Build history of the part. All positions in model axes, mm. A direction names the side the tool comes from. Round coordinates to 2 decimals unless told otherwise and drop trailing zeros. Loops run counter-clockwise (first coordinate to the right, second up) from the corner with the lowest first, then second, coordinate; pieces in that order, holes last. Notation, with made-up numbers: M 58,0.5 L 71,0.5 A17 ccw 71,33.5 Z; hole C -15,-33.75 d4. An arc over 180 degrees is marked long. One line per item, written item: value.
```python
from build123d import *

# Parameters (mm, degrees)
SKETCH1_R           = 38.1
SKETCH1_R_2         = 6.35
BOSS_EXTRUDE1_DEPTH = 2.54
SKETCH2_R           = 8.89
SKETCH2_R_2         = 6.35
BOSS_EXTRUDE2_DEPTH = 6.35
SKETCH5_R           = 38.1
SKETCH5_R_2         = 30.48
BOSS_EXTRUDE3_DEPTH = 2.54
SKETCH6_R           = 38.1
SKETCH6_R_2         = 35.56
BOSS_EXTRUDE4_DEPTH = 6.35


with BuildPart() as part:
    # Sketch1 → Boss-Extrude1 (new body)
    with BuildSketch(Plane(origin=(0, 0, 0), x_dir=(1, 0, 0), z_dir=(0, 1, 0))):
        with Locations(Location((0, 0, 0), (0, 0, 270))):
            Circle(SKETCH1_R)
        with Locations(Location((0, 0, 0), (0, 0, 270))):
            Circle(SKETCH1_R_2, mode=Mode.SUBTRACT)
    extrude(amount=BOSS_EXTRUDE1_DEPTH)

    # Sketch2 → Boss-Extrude2 (add)
    with BuildSketch(Plane(origin=(0, 2.54, 0), x_dir=(1, 0, 0), z_dir=(0, 1, 0))):
        with Locations(Location((0, 0, 0), (0, 0, 270))):
            Circle(SKETCH2_R)
        with Locations(Location((0, 0, 0), (0, 0, 270))):
            Circle(SKETCH2_R_2, mode=Mode.SUBTRACT)
    extrude(amount=BOSS_EXTRUDE2_DEPTH)

    # Sketch5 → Boss-Extrude3 (add)
    with BuildSketch(Plane(origin=(0, 2.54, 0), x_dir=(1, 0, 0), z_dir=(0, 1, 0))):
        with Locations(Location((0, 0, 0), (0, 0, 270))):
            Circle(SKETCH5_R)
        with Locations(Location((0, 0, 0), (0, 0, 270))):
            Circle(SKETCH5_R_2, mode=Mode.SUBTRACT)
    extrude(amount=BOSS_EXTRUDE3_DEPTH)

    # Sketch6 → Boss-Extrude4 (add)
    with BuildSketch(Plane(origin=(0, 5.08, 0), x_dir=(1, 0, 0), z_dir=(0, 1, 0))):
        with Locations(Location((0, 0, 0), (0, 0, 270))):
            Circle(SKETCH6_R)
        with Locations(Location((0, 0, 0), (0, 0, 270))):
            Circle(SKETCH6_R_2, mode=Mode.SUBTRACT)
    extrude(amount=BOSS_EXTRUDE4_DEPTH)


solid = part.part
```
Item 1: Slice it at D-D, the plane y = 1.25. Give the cut face in (x, z), and give its area (3 significant figures).
Check values:
outline: C 0,0 d76.2; hole C 0,0 d12.7
area: 4,430 mm2
Item 2: Pull direction X, two halves, no side cores. Call faces 1 (the face through (-23.183, 5.635, -30.235)), 2 (the face through (30.22, 3.79, -3.97)), 3 (the face through (11, 11.43, 34)): pulls with the +X half, pulls with the -X half, needs draft (parallel to the pull), parting line crosses it, or undercut.
Check values:
face 1: parting line crosses it
face 2: undercut
face 3: needs draft
Item 3: Drop flat-ended pins along their axis: P1, Ø14.5, axis at x = 0, z = 0, coming from the +Y side; P2, Ø2, axis at x = -1.5, z = 10, coming from the +Y side; P3, Ø12, axis at x = 17.5, z = 20, coming from the +Y side. Give the stop position or say it passes through.
Check values:
P1: stops at y = 8.89
P2: stops at y = 2.54
P3: stops at y = 5.08
Item 4: Slice it at A-A, the plane x = 0. Give the cut face in (y, z).
Check values:
outline: M 0,-38.1 L 11.43,-38.1 L 11.43,-35.56 L 5.08,-35.56 L 5.08,-30.48 L 2.54,-30.48 L 2.54,-8.89 L 8.89,-8.89 L 8.89,-6.35 L 0,-6.35 Z; M 0,6.35 L 8.89,6.35 L 8.89,8.89 L 2.54,8.89 L 2.54,30.48 L 5.08,30.48 L 5.08,35.56 L 11.43,35.56 L 11.43,38.1 L 0,38.1 Z
Item 5: Wall check: line 1 along X through (y, z) = (8.25, 0); line 2 along X through (y, z) = (3.35, 0); line 3 along X through (y, z) = (9.25, 0). Give the ranges that are in metal, low to high.
Check values:
line 1: x = -38.1 to -35.56, -8.89 to -6.35, 6.35 to 8.89, 35.56 to 38.1
line 2: x = -38.1 to -30.48, -8.89 to -6.35, 6.35 to 8.89, 30.48 to 38.1
line 3: x = -38.1 to -35.56, 35.56 to 38.1
Item 6: Slice it at C-C, the plane y = 8. Give the cut face in (x, z).
Check values:
outline: C 0,0 d76.2; C 0,0 d17.78; hole C 0,0 d71.12; hole C 0,0 d12.7
Item 7: Which spindle directions (+Z, -Z, +X, -X, +Y, -Y) get a long thin tool onto all of the face, cutting with end or side? Do faces 4 (the face through (-8.68, 5.67, -1.93)), 5 (the face through (-3.86, 4.38, -5.04)). Say none if no direction does.
Check values:
face 4: +Y
face 5: +Y, -Y
Item 8: Slice it at B-B, the plane z = 0. Give the cut face in (x, y), and give its area (3 significant figures).
Check values:
outline: M -38.1,0 L -6.35,0 L -6.35,8.89 L -8.89,8.89 L -8.89,2.54 L -30.48,2.54 L -30.48,5.08 L -35.56,5.08 L -35.56,11.43 L -38.1,11.43 Z; M 6.35,0 L 38.1,0 L 38.1,11.43 L 35.56,11.43 L 35.56,5.08 L 30.48,5.08 L 30.48,2.54 L 8.89,2.54 L 8.89,8.89 L 6.35,8.89 Z
area: 265 mm2
